Read the model definition and answer for the solid it produces. Units are mm, in the model's axes. Face numbers are marked on the shaded views. A direction names the side the tool comes from. Give positions to 0.01 mm unless a question says otherwise; leave off trailing zeros. Loops run counter-clockwise (first coordinate to the right, second up) from the corner with the lowest first, then second, coordinate; pieces in that order, holes last. Notation, with made-up numbers: (40.25, 43.25) - (65.25, 43.25) arc R35 ccw to (65.25, 77.25) - close; hole circle Ø2 at (36.25, 88.5). An arc over 180 degrees is marked (long way). Use a Markdown table: item, result. Add a question column.
Item 1: Consider probe 1 along Y at (x, z) = (-5.5, 22.25); probe 2 along Z at (x, y) = (-11, -6); probe 3 along Z at (x, y) = (5.75, 11.25). Determine where each line is inside the solid, lowest interval first. Write a range as [from, to].
Item 2: Each of these flat-tipped pins is pushed along its axis until it touches: P1, Ø1.5, axis at x = -2.5, y = 0.5, coming from the -Z side; P2, Ø1.5, axis at y = -0.5, z = 11, coming from the -X side; P3, Ø1.5, axis at x = -3, z = 19, coming from the -Y side; P4, Ø8, axis at y = -0.5, z = 20.5, coming from the +X side. Where does it stop, or does it pass through?
Item 3: A cutting plane is placed at A-A (y = 4). Determine the outline of the cut face in (x, z), plus the area to 3 significant figures.
Item 4: Which of the six approach directions +Z, -Z, +X, -X, +Y, -Y give full straight-line access (tool end or side, diameter ignored) to the marked faces 1, 2, 3, 4 and 5?
Item 5: A cutting plane is placed at C-C (z = 19.25). Determine the outline of the cut face in (x, y).
Item 6: A cutting plane is placed at D-D (z = 8.5). Determine the outline of the cut face in (x, y), plus the area to 3 significant figures.
Item 7: A cutting plane is placed at B-B (x = -1.75). Determine the outline of the cut face in (y, z), plus the area to 3 significant figures.
from build123d import *

# Parameters (mm, degrees)
F1_DEPTH = 20.32
F2_DEPTH = 15.24
F3_DEPTH = 25.4
F4_DEPTH = 10.16
F5_DEPTH = 5.08


with BuildPart() as f1:
    # F0 (on Top) → F1 (new body)
    with BuildSketch(Plane.XY):
        with BuildLine():
            Line((-0.715326, 13.86313), (-10.875326, 13.86313))
            ThreePointArc((-10.875326, 13.86313), (-12.671377, 13.119181), (-13.415326, 11.32313))
            Line((-13.415326, 11.32313), (-13.415326, 1.16313))
            Line((-13.415326, 1.16313), (-5.795326, 1.16313))
            Line((-5.795326, 1.16313), (-5.795326, 6.24313))
            Line((-5.795326, 6.24313), (-0.715326, 6.24313))
            Line((-0.715326, 6.24313), (-0.715326, 13.86313))
        make_face()
    extrude(amount=F1_DEPTH)

    # F0 (on Top) → F2 (join)
    with BuildSketch(Plane.XY):
        with BuildLine():
            Line((9.444674, 13.86313), (-0.715326, 13.86313))
            Line((-0.715326, 13.86313), (-0.715326, 6.24313))
            Line((-0.715326, 6.24313), (4.364674, 6.24313))
            Line((4.364674, 6.24313), (4.364674, 1.16313))
            Line((4.364674, 1.16313), (11.984674, 1.16313))
            Line((11.984674, 1.16313), (11.984674, 11.32313))
            ThreePointArc((11.984674, 11.32313), (11.240725, 13.119181), (9.444674, 13.86313))
        make_face()
    extrude(amount=F2_DEPTH)

    # F0 (on Top) → F3 (join)
    with BuildSketch(Plane.XY):
        Polygon((4.364674, 6.24313), (-0.715326, 6.24313), (-5.795326, 6.24313), (-5.795326, 1.16313), (-5.795326, -3.91687), (-0.715326, -3.91687), (4.364674, -3.91687), (4.364674, 1.16313), align=None)
    extrude(amount=F3_DEPTH)

    # F0 (on Top) → F4 (join)
    with BuildSketch(Plane.XY):
        with BuildLine():
            Line((11.984674, -8.99687), (11.984674, 1.16313))
            Line((11.984674, 1.16313), (4.364674, 1.16313))
            Line((4.364674, 1.16313), (4.364674, -3.91687))
            Line((4.364674, -3.91687), (-0.715326, -3.91687))
            Line((-0.715326, -3.91687), (-0.715326, -11.53687))
            Line((-0.715326, -11.53687), (9.444674, -11.53687))
            ThreePointArc((9.444674, -11.53687), (11.240725, -10.792922), (11.984674, -8.99687))
        make_face()
    extrude(amount=F4_DEPTH)

    # F0 (on Top) → F5 (join)
    with BuildSketch(Plane.XY):
        with BuildLine():
            Line((-5.795326, 1.16313), (-13.415326, 1.16313))
            Line((-13.415326, 1.16313), (-13.415326, -8.99687))
            ThreePointArc((-13.415326, -8.99687), (-12.671377, -10.792922), (-10.875326, -11.53687))
            Line((-10.875326, -11.53687), (-0.715326, -11.53687))
            Line((-0.715326, -11.53687), (-0.715326, -3.91687))
            Line((-0.715326, -3.91687), (-5.795326, -3.91687))
            Line((-5.795326, -3.91687), (-5.795326, 1.16313))
        make_face()
    extrude(amount=F5_DEPTH)


solid = f1.part
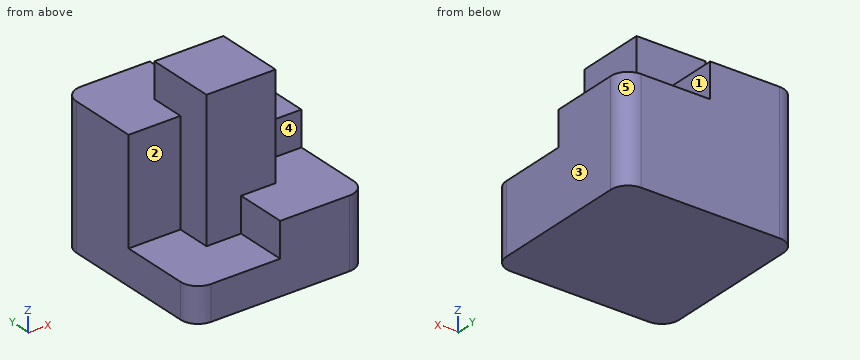
Geometry says:
| question | item | result |
|---|---|---|
| 1 | probe 1 | [-3.92, 6.24] |
| 1 | probe 2 | [0, 5.08] |
| 1 | probe 3 | [0, 15.24] |
| 2 | P1 | z = 0 |
| 2 | P2 | x = -5.8 |
| 2 | P3 | y = -3.92 |
| 2 | P4 | x = 4.36 |
| 3 | outline | (-13.42, 0) - (11.98, 0) - (11.98, 15.24) - (4.36, 15.24) - (4.36, 25.4) - (-5.8, 25.4) - (-5.8, 20.32) - (-13.42, 20.32) - close |
| 3 | area | 529 mm² |
| 4 | face 1 | +Z, +X, +Y |
| 4 | face 2 | +Z, -X, -Y |
| 4 | face 3 | +Z, -Z, +X, +Y, -Y |
| 4 | face 4 | +Z, +X, -Y |
| 4 | face 5 | +Z, -Z, +X, +Y |
| 5 | outline | (-13.42, 1.16) - (-5.8, 1.16) - (-5.8, -3.92) - (4.36, -3.92) - (4.36, 6.24) - (-0.72, 6.24) - (-0.72, 13.86) - (-10.88, 13.86) arc R2.54 ccw to (-13.42, 11.32) - close |
| 6 | outline | (-13.42, 1.16) - (-5.8, 1.16) - (-5.8, -3.92) - (-0.72, -3.92) - (-0.72, -11.54) - (9.44, -11.54) arc R2.54 ccw to (11.98, -9) - (11.98, 11.32) arc R2.54 ccw to (9.44, 13.86) - (-10.88, 13.86) arc R2.54 ccw to (-13.42, 11.32) - close |
| 6 | area | 506 mm² |
| 7 | outline | (-11.54, 0) - (13.86, 0) - (13.86, 20.32) - (6.24, 20.32) - (6.24, 25.4) - (-3.92, 25.4) - (-3.92, 5.08) - (-11.54, 5.08) - close |
| 7 | area | 452 mm² |
